Work out the finished part from the listing and answer in its coordinate system (mm). A direction names the side the tool comes from. Give positions to 0.01 mm unless a question says otherwise; leave off trailing zeros. Loops run counter-clockwise (first coordinate to the right, second up) from the corner with the lowest first, then second, coordinate; pieces in that order, holes last. Notation, with made-up numbers: M -13.5,60 L 43.5,60 A4 cw 43.5,67 Z; hole C 84,8.5 d4. An arc over 180 degrees is marked long. Use a Markdown table: item, result.
```python
from build123d import *

# Parameters (mm, degrees)
F0_W     = 76.187346
F0_H     = 152.374692
F1_DEPTH = 7.112
F2_R     = 5.08
F3_R     = 1.524
F4_T     = -0.762
F5_W     = 7.632177
F5_H     = 7.64653
F6_DEPTH = 25.4
F7_R     = 1.524
F8_W     = 7.637478
F8_H     = 3.121578
F9_DEPTH = 25.4
F10_R    = 1.016


with BuildPart() as f1:
    # F0 (on Top) → F1 (new body)
    with BuildSketch(Plane.XY):
        with Locations((2.484182, -2.768833)):
            Rectangle(F0_W, F0_H)
    extrude(amount=F1_DEPTH)

    # F2
    f2_edges = [f1.edges().sort_by_distance(p)[0] for p in [
        (40.577855, -78.956179, 3.556),
        (-35.609491, -78.956179, 3.556),
        (-35.609491, 73.418513, 3.556),
        (40.577855, 73.418513, 3.556),
    ]]
    fillet(f2_edges, radius=F2_R)

    # F3
    f3_edges = [f1.edges().sort_by_distance(p)[0] for p in [
        (40.577855, -2.768833, 7.112),
        (-35.609491, -2.768833, 7.112),
    ]]
    fillet(f3_edges, radius=F3_R)

    # F4
    f4_openings = [f1.faces().sort_by_distance(p)[0] for p in [
        (2.484182, -2.768833, 0),
    ]]
    offset(amount=F4_T, openings=f4_openings)

    # F5 (on face) → F6 (cut)
    with BuildSketch(Plane.XY.offset(7.112)):
        with Locations((-26.713403, 64.515248)):
            Rectangle(F5_W, F5_H)
    extrude(amount=-F6_DEPTH, mode=Mode.SUBTRACT)

    # F7
    f7_edges = [f1.edges().sort_by_distance(p)[0] for p in [
        (-22.897314, 60.691983, 6.731),
        (-30.529491, 60.691983, 6.731),
        (-22.897314, 68.338513, 6.731),
        (-30.529491, 68.338513, 6.731),
    ]]
    fillet(f7_edges, radius=F7_R)

    # F8 (on face) → F9 (cut)
    with BuildSketch(Plane.XY.offset(7.112)):
        with Locations((-26.710752, 55.848118)):
            Rectangle(F8_W, F8_H)
    extrude(amount=-F9_DEPTH, mode=Mode.SUBTRACT)

    # F10
    f10_edges = [f1.edges().sort_by_distance(p)[0] for p in [
        (-30.529491, 54.287329, 6.731),
        (-22.892013, 54.287329, 6.731),
        (-30.529491, 57.408907, 6.731),
        (-22.892013, 57.408907, 6.731),
    ]]
    fillet(f10_edges, radius=F10_R)


solid = f1.part
```
(1) Consider probe 1 along X at (y, z) = (-63, 2.25); probe 2 along Y at (x, z) = (-22.5, 0.5); probe 3 along Z at (x, y) = (-15.5, 59.5). Determine where each line is inside the solid, lowest interval first. Write a range as [from, to].
Entries:
| item | result |
|---|---|
| probe 1 | x = [-35.61, -34.85], [39.82, 40.58] |
| probe 2 | y = [-78.96, -78.19], [72.66, 73.42] |
| probe 3 | z = [6.35, 7.11] |
(2) Given P1, Ø0.6, axis at x = -25.5, z = 7, coming from the -Y side; P2, Ø0.6, axis at x = -26.5, z = 7, coming from the +Y side; P3, Ø22, axis at x = -4, y = 4, coming from the -Z side, each flat-ended and moving along its own axis, determine where each tip first touches the part or whether it passes through.
Entries:
| item | result |
|---|---|
| P1 | stops at y = -78.47 |
| P2 | stops at y = 72.94 |
| P3 | stops at z = 6.35 |
(3) A cutting plane is placed at A-A (z = 3.75). Write down the section's boundary in (x, y), and give its area (3 significant figures).
Entries:
| item | result |
|---|---|
| outline | M -35.61,-73.88 A5.08 ccw -30.53,-78.96 L 35.5,-78.96 A5.08 ccw 40.58,-73.88 L 40.58,68.34 A5.08 ccw 35.5,73.42 L -30.53,73.42 A5.08 ccw -35.61,68.34 Z; hole M -34.85,-73.88 A4.32 ccw -30.53,-78.19 L 35.5,-78.19 A4.32 ccw 39.82,-73.88 L 39.82,68.34 A4.32 ccw 35.5,72.66 L -30.53,72.66 A4.32 ccw -34.85,68.34 Z |
| area | 340 mm² |
(4) Which of the six approach directions +Z, -Z, +X, -X, +Y, -Y give full straight-line access (tool end or side, diameter ignored) to faces 1 (the cylindrical face through (38.58, 71.36, 2.83)), 2 (the cylindrical face through (39.13, 71.89, 2.83))?
Entries:
| item | result |
|---|---|
| face 1 | -Z |
| face 2 | +Z, -Z, +X, +Y |
(5) A cutting plane is placed at C-C (y = 48). Write down the section's boundary in (x, z), and give its area (3 significant figures).
Entries:
| item | result |
|---|---|
| outline | M -35.61,0 L -34.85,0 L -34.85,5.59 A0.76 cw -34.09,6.35 L 39.05,6.35 A0.76 cw 39.82,5.59 L 39.82,0 L 40.58,0 L 40.58,5.59 A1.52 ccw 39.05,7.11 L -34.09,7.11 A1.52 ccw -35.61,5.59 Z |
| area | 67.0 mm² |
(6) A cutting plane is placed at B-B (x = -2). Write down the section's boundary in (y, z), and give its area (3 significant figures).
Entries:
| item | result |
|---|---|
| outline | M -78.96,0 L -78.19,0 L -78.19,5.59 A0.76 cw -77.43,6.35 L 71.89,6.35 A0.76 cw 72.66,5.59 L 72.66,0 L 73.42,0 L 73.42,5.59 A1.52 ccw 71.89,7.11 L -77.43,7.11 A1.52 ccw -78.96,5.59 Z |
| area | 125 mm² |
(7) The mould has two halves that part along X. Classify faces 3 (the cylindrical face through (38.52, -76.96, 2.83)), 4 (the cylindrical face through (-34.16, -77.43, 2.83)), 5 (the flat face through (2, 73.419, 3)): released by +X, released by -X, zero draft, split by the parting line, or undercut.
Entries:
| item | result |
|---|---|
| face 3 | undercut |
| face 4 | released by -X |
| face 5 | zero draft |
